```python
from build123d import *

# Parameters (mm, degrees)
F0_R     = 60
F1_DEPTH = 7.5
F2_R     = 60
F2_R_2   = 52.5
F3_DEPTH = 75
F4_R     = 56.25
F5_DEPTH = 5


with BuildPart() as f1:
    # F0 (on Top) → F1 (new body)
    with BuildSketch(Plane.XY):
        Circle(F0_R)
    extrude(amount=F1_DEPTH)

    # F2 (on face) → F3 (join)
    with BuildSketch(Plane.XY.offset(7.5)):
        Circle(F2_R)
        Circle(F2_R_2, mode=Mode.SUBTRACT)
    extrude(amount=F3_DEPTH)

    # F4 (on face) → F5 (cut)
    with BuildSketch(Plane.XY.offset(82.5)):
        Circle(F4_R)
    extrude(amount=-F5_DEPTH, mode=Mode.SUBTRACT)


solid = f1.part
```
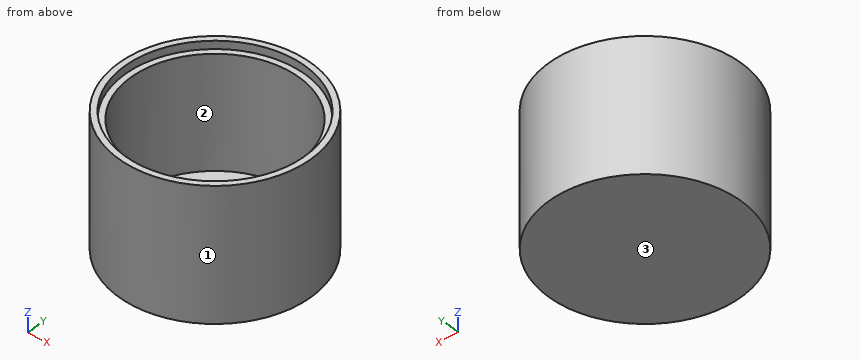
Build history of the part. All positions in model axes, mm. Face numbers are marked on the shaded views. Give positions to 0.01 mm unless a question says otherwise; leave off trailing zeros. Order: outer loops, then holes, each group sorted by start corner. A loop starts at its lowest first (then second) coordinate and runs counter-clockwise, first axis right, second up. Notation, with made-up numbers: M -14,47.25 L 16,47.25 A36 cw 16,83.25 Z; hole C 87,67 d1. An arc over 180 degrees is marked long. Return JSON: item names as keys, results as strings.
Q1. Two-plate mould, pull along Y, no slides. Class the marked faces 1, 2 and 3: pulls with the +Y half, pulls with the -Y half, needs draft (parallel to the pull), parting line crosses it, or undercut.
Answer list:
{"face 1": "parting line crosses it", "face 2": "undercut", "face 3": "needs draft"}
Q2. Flat gauge pins, fed straight in: pin 1 (1.5 mm diameter, centred on x = -15.5, z = 58, fed in from -Y); pin 2 (1 mm diameter, centred on y = 13.5, z = 55, fed in from -X); pin 3 (12 mm diameter, centred on x = 33.5, z = 66.5, fed in from +Y). Where does each tip first touch, or does it go through?
Answer list:
{"pin 1": "stops at y = -58.16", "pin 2": "stops at x = -58.57", "pin 3": "stops at y = 53.33"}
Q3. Wall check: probe 1 along Y at (x, z) = (0, 79); probe 2 along X at (y, z) = (-1.5, 29.5); probe 3 along Y at (x, z) = (0, 51.5). Give the ranges that are in metal, low to high. Write a range as from..to.
Answer list:
{"probe 1": "y = -60..-56.25, 56.25..60", "probe 2": "x = -59.98..-52.48, 52.48..59.98", "probe 3": "y = -60..-52.5, 52.5..60"}
Q4. Band-saw the part on A-A (y = 0). Give the cut face in (x, z).
Answer list:
{"outline": "M -60,0 L 60,0 L 60,82.5 L 56.25,82.5 L 56.25,77.5 L 52.5,77.5 L 52.5,7.5 L -52.5,7.5 L -52.5,77.5 L -56.25,77.5 L -56.25,82.5 L -60,82.5 Z"}
Q5. Band-saw the part on B-B (z = 74.5). Give the cut face in (x, y), then the cut area to 3 significant figures.
Answer list:
{"outline": "C 0,0 d120; hole C 0,0 d105", "area": "2,650 mm^2"}
